```python
from build123d import *
from build123d.topology import SkipClean

# Parameters (mm, degrees)
BOSS_EXTRUDE1_DEPTH = 2.5
SKETCH3_R           = 1.5
BOSS_EXTRUDE2_DEPTH = 3


with BuildPart() as part:
    # Sketch1 → Boss-Extrude1 (new body)
    # profile 1 of 2: a face of its own
    with BuildSketch(Plane.XY):
        with BuildLine():
            ThreePointArc((-7.542881817, 0.082245335), (-0.042881817, -7.417754665), (7.457118183, 0.082245335))
            ThreePointArc((7.457118183, 0.082245335), (-0.042881817, 7.582245335), (-7.542881817, 0.082245335))
        make_face()
        Polygon((1.632118183, 2.983430437), (3.307118183, 0.082245335), (1.632118183, -2.818939768), (-0.042881817, -2.818939768), (-1.717881817, -2.818939768), (-3.392881817, 0.082245335), (-1.717881817, 2.983430437), (-0.042881817, 2.983430437), align=None, mode=Mode.SUBTRACT)
    # profile 2 of 2: a face of its own
    with BuildSketch(Plane.XY):
        with BuildLine():
            Line((7.457118183, -33.176547175), (7.457118183, 0.082245335))
            ThreePointArc((7.457118183, 0.082245335), (-0.042881817, -7.417754665), (-7.542881817, 0.082245335))
            Line((-7.542881817, 0.082245335), (-7.542881817, -33.176547175))
            Line((-7.542881817, -33.176547175), (7.457118183, -33.176547175))
        make_face()
    extrude(amount=BOSS_EXTRUDE1_DEPTH)

    # Sketch3 → Boss-Extrude2 (add)
    with SkipClean():  # the faces are left unmerged after this step: merging them gives an invalid solid
        with BuildSketch(Plane.XY.offset(2.5)):
            with BuildLine():
                Line((7.457118183, 0.082245335), (7.457118183, -33.176547175))
                Line((7.457118183, -33.176547175), (-7.542881817, -33.176547175))
                Line((-7.542881817, -33.176547175), (-7.542881817, 0.082245335))
                ThreePointArc((-7.542881817, 0.082245335), (-0.042881817, 7.582245335), (7.457118183, 0.082245335))
            make_face()
            with Locations((-0.042881817, 0.082245335)):
                Circle(SKETCH3_R, mode=Mode.SUBTRACT)
        extrude(amount=BOSS_EXTRUDE2_DEPTH)
    add(part.part.scale(1), mode=Mode.REPLACE)  # the faces are merged on a copy


solid = part.part
```
Here's how the part is built. I have some questions about the finished solid (model axes, mm). A direction names the side the tool comes from. Give positions to 0.01 mm unless a question says otherwise; leave off trailing zeros. Order: outer loops, then holes, each group sorted by start corner. A loop starts at its lowest first (then second) coordinate and runs counter-clockwise, first axis right, second up. Notation, with made-up numbers: (50.5, 30) - (105.5, 30) arc R15 ccw to (105.5, 58) - close; hole circle Ø9 at (89.5, 22.25). An arc over 180 degrees is marked (long way). Answer as a JSON object with one key per item and string values. Group by question number.
Item 1: For P1, Ø1.5, axis at x = -4, z = 1, coming from the +Y side; P2, Ø2, axis at x = 0.5, z = 1.5, coming from the +Y side; P3, Ø1.5, axis at x = 1.5, z = 1.5, coming from the +Y side, each with a flat end and sliding along its axis, tell me the tip position at first contact or that it passes through.
Item 2: If we section it at A-A on z = 0.75: Please give me the cut outline in (x, y), and give its area (3 significant figures).
Item 3: Please list where these lines run through material, in increasing order: probe 1 along Y at (x, z) = (0.25, 2.45); probe 2 along X at (y, z) = (-1.5, 1.4); probe 3 along Y at (x, z) = (0.75, 3.1).
Item 4: If we section it at D-D on y = 4: Please give me the cut outline in (x, z).
Item 5: If we section it at B-B on x = 1: Please give me the cut outline in (y, z), and give its area (3 significant figures).
Item 6: If we mould it in two halves opening along Y, with no side actions, what happens to faces 1 (the flat face through (7.457, -16, 3)), 2 (the flat face through (1.5, 0.8, 2.5)), 3 (the cylindrical face through (-0.21, 7.58, 2.71))? For each: pulls with the +Y half, pulls with the -Y half, needs draft (parallel to the pull), parting line crosses it, or undercut.
Item 7: Which directions (+Z, -Z, +X, -X, +Y, -Y) give clear straight access to the entire face, cutting with the end or side of a thin tool? Please do faces 4 (the flat face through (-7.543, -17, 3)), 5 (the flat face through (0, -2.819, 1)).
Item 8: If we section it at C-C on z = 3.15: Please give me the cut outline in (x, y).
Result set:
{
 "1": {"P1": "y = 6.86", "P2": "y = 7.58", "P3": "y = 7.54"},
 "2": {"outline": "(-7.54, -33.18) - (7.46, -33.18) - (7.46, 0.08) arc R7.5 ccw to (-7.54, 0.08) - close; hole (-3.39, 0.08) - (-1.72, -2.82) - (1.63, -2.82) - (3.31, 0.08) - (1.63, 2.98) - (-1.72, 2.98) - close", "area": "558 mm²"},
 "3": {"probe 1": "-33.18 to -2.82, 2.98 to 7.58", "probe 2": "-7.54 to -2.48, 2.39 to 7.46", "probe 3": "-33.18 to -1.19, 1.36 to 7.54"},
 "4": {"outline": "(-6.44, 0) - (6.35, 0) - (6.35, 5.5) - (-6.44, 5.5) - close"},
 "5": {"outline": "(-33.18, 0) - (-2.82, 0) - (-2.82, 2.5) - (-1, 2.5) - (-1, 5.5) - (-33.18, 5.5) - close; (1.16, 2.5) - (2.98, 2.5) - (2.98, 0) - (7.51, 0) - (7.51, 5.5) - (1.16, 5.5) - close", "area": "203 mm²"},
 "6": {"face 1": "needs draft", "face 2": "undercut", "face 3": "pulls with the +Y half"},
 "7": {"face 4": "+Z, -Z, -X, +Y, -Y", "face 5": "-Z"},
 "8": {"outline": "(-7.54, -33.18) - (7.46, -33.18) - (7.46, 0.08) arc R7.5 ccw to (-7.54, 0.08) - close; hole circle Ø3 at (-0.04, 0.08)"}
}
